from build123d import *

# Parameters (mm, degrees)
SKETCH1_W           = 75
SKETCH1_H           = 148
BOSS_EXTRUDE1_DEPTH = 10
SKETCH2_W           = 55
SKETCH2_H           = 8
BOSS_EXTRUDE2_DEPTH = 42
SKETCH3_W           = 26.5
SKETCH3_H           = 24
CUT_EXTRUDE1_DEPTH  = 8
SKETCH4_W           = 8
SKETCH4_H           = 30
SKETCH4_H_2         = 25
BOSS_EXTRUDE3_DEPTH = 42
SKETCH5_R           = 2.5
CUT_EXTRUDE2_DEPTH  = 8
CUT_EXTRUDE3_DEPTH  = 8
SKETCH10_R          = 2.75
CUT_EXTRUDE5_DEPTH  = 10
SKETCH11_W          = 47
SKETCH11_H          = 85
CUT_EXTRUDE6_DEPTH  = 10


with BuildPart() as part:
    # Sketch1 → Boss-Extrude1 (new body)
    with BuildSketch(Plane.XY):
        with Locations((27.5, -70)):
            Rectangle(SKETCH1_W, SKETCH1_H)
    extrude(amount=BOSS_EXTRUDE1_DEPTH)

    # Sketch2 → Boss-Extrude2 (add)
    with BuildSketch(Plane.XY.offset(10)):
        with Locations((37.5, -115)):
            Rectangle(SKETCH2_W, SKETCH2_H)
    extrude(amount=BOSS_EXTRUDE2_DEPTH)

    # Sketch3 → Cut-Extrude1 (cut)
    with BuildSketch(Plane(origin=(0, -119, 0), x_dir=(-1, 0, 0), z_dir=(0, -1, 0))):
        with Locations((-34.85, -31.15)):
            Rectangle(SKETCH3_W, SKETCH3_H)
    extrude(amount=-CUT_EXTRUDE1_DEPTH, mode=Mode.SUBTRACT)

    # Sketch4 → Boss-Extrude3 (add)
    with BuildSketch(Plane.XY.offset(10)):
        with Locations((61, -11)):
            Rectangle(SKETCH4_W, SKETCH4_H)
        with Locations((61, -131.5)):
            Rectangle(SKETCH4_W, SKETCH4_H_2)
    extrude(amount=BOSS_EXTRUDE3_DEPTH)

    # Sketch5 → Cut-Extrude2 (cut)
    with BuildSketch(Plane.ZY.offset(-57)):
        with Locations((18, -11)):
            Circle(SKETCH5_R)
        with Locations((44, -11)):
            Circle(SKETCH5_R)
        with Locations((44, -129)):
            Circle(SKETCH5_R)
        with Locations((18, -129)):
            Circle(SKETCH5_R)
    extrude(amount=-CUT_EXTRUDE2_DEPTH, mode=Mode.SUBTRACT)

    # Sketch6 → Cut-Extrude3 (cut)
    with BuildSketch(Plane(origin=(0, -119, 0), x_dir=(-1, 0, 0), z_dir=(0, -1, 0))):
        with BuildLine():
            Line((-19.4, -45.1), (-17.4, -45.1))
            ThreePointArc((-17.4, -45.1), (-15.85, -46.65), (-17.4, -48.2))
            Line((-17.4, -48.2), (-19.4, -48.2))
            ThreePointArc((-19.4, -48.2), (-20.95, -46.65), (-19.4, -45.1))
        make_face()
        with BuildLine():
            Line((-19.4, -14.1), (-17.4, -14.1))
            ThreePointArc((-17.4, -14.1), (-15.85, -15.65), (-17.4, -17.2))
            Line((-17.4, -17.2), (-19.4, -17.2))
            ThreePointArc((-19.4, -17.2), (-20.95, -15.65), (-19.4, -14.1))
        make_face()
        with BuildLine():
            Line((-50.4, -45.1), (-48.4, -45.1))
            ThreePointArc((-48.4, -45.1), (-46.85, -46.65), (-48.4, -48.2))
            Line((-48.4, -48.2), (-50.4, -48.2))
            ThreePointArc((-50.4, -48.2), (-51.95, -46.65), (-50.4, -45.1))
        make_face()
        with BuildLine():
            Line((-50.4, -14.1), (-48.4, -14.1))
            ThreePointArc((-48.4, -14.1), (-46.85, -15.65), (-48.4, -17.2))
            Line((-48.4, -17.2), (-50.4, -17.2))
            ThreePointArc((-50.4, -17.2), (-51.95, -15.65), (-50.4, -14.1))
        make_face()
    extrude(amount=-CUT_EXTRUDE3_DEPTH, mode=Mode.SUBTRACT)

    # Sketch10 → Cut-Extrude5 (cut)
    with BuildSketch(Plane(origin=(0, 0, 0), x_dir=(-1, 0, 0), z_dir=(0, 0, -1))):
        with Locations((-1, -102.8)):
            Circle(SKETCH10_R)
        with Locations((-1, -134.8)):
            Circle(SKETCH10_R)
        with Locations((-1, -37.7)):
            Circle(SKETCH10_R)
        with Locations((-1, -5.7)):
            Circle(SKETCH10_R)
    extrude(amount=-CUT_EXTRUDE5_DEPTH, mode=Mode.SUBTRACT)

    # Sketch11 → Cut-Extrude6 (cut)
    with BuildSketch(Plane(origin=(0, 0, 0), x_dir=(-1, 0, 0), z_dir=(0, 0, -1))):
        with Locations((-41.5, -67.5)):
            Rectangle(SKETCH11_W, SKETCH11_H)
    extrude(amount=-CUT_EXTRUDE6_DEPTH, mode=Mode.SUBTRACT)


solid = part.part
Verification items for the finished model (mm, model axes). A direction names the side the tool comes from. Coordinates: 2 decimals unless noted, no trailing zeros. Order: outer loops, then holes, each group sorted by start corner. A loop starts at its lowest first (then second) coordinate and runs counter-clockwise, first axis right, second up.
Item 1: Material ranges on L1, parallel to Y at x = 62.25, z = 44; L2, parallel to Z at x = 61, y = -129; L3, parallel to Z at x = 37, y = -124, recorded low to high.
Filled in:
L1: y = -144 to -131.5, -126.5 to -111, -26 to -13.5, -8.5 to 4
L2: z = 0 to 15.5, 20.5 to 41.5, 46.5 to 52
L3: z = 0 to 10
Item 2: Release check for a two-part mould opening along Y. For faces 1 (the face through (38, 4, 9)), 2 (the face through (20.95, -115.06, 46.68)), 3 (the face through (60.94, -11.96, 46.31)) record: +Y half, -Y half, draft (parallel to the pull), parting line (faces both ways), or undercut.
Filled in:
face 1: +Y half
face 2: draft
face 3: undercut
Item 3: Section check C-C, the plane z = 26.5. Enter the section's corners in (x, y), then the cut area to 3 significant figures.
Filled in:
outline: (10, -119) - (21.6, -119) - (21.6, -111) - (10, -111) - close; (48.1, -119) - (57, -119) - (57, -144) - (65, -144) - (65, -111) - (48.1, -111) - close; (57, -26) - (65, -26) - (65, 4) - (57, 4) - close
area: 668 mm2
Item 4: Depth check by flat-ended pin: pin 1 (2 mm diameter, centred on x = 49.5, y = -113, fed in from -Z); pin 2 (12.5 mm diameter, centred on y = -132, z = 25.5, fed in from -X); pin 3 (4 mm diameter, centred on x = 18, y = -33, fed in from +Z); pin 4 (6.5 mm diameter, centred on y = -116.5, z = 38.5, fed in from -X). Enter the tip coordinate at first touch or a pass-through.
Filled in:
pin 1: stops at z = 0
pin 2: stops at x = 57
pin 3: stops at z = 10
pin 4: stops at x = 10
Item 5: Section check A-A, the plane x = 59.5. Enter the section's corners in (y, z), then the cut area to 3 significant figures.
Filled in:
outline: (-144, 0) - (-110, 0) - (-110, 10) - (-111, 10) - (-111, 52) - (-144, 52) - close; (-26, 10) - (-25, 10) - (-25, 0) - (4, 0) - (4, 52) - (-26, 52) - close; hole circle Ø5 at (-129, 18); hole circle Ø5 at (-129, 44); hole circle Ø5 at (-11, 18); hole circle Ø5 at (-11, 44)
area: 3,200 mm2
Item 6: Section check D-D, the plane x = 1. Enter the section's corners in (y, z).
Filled in:
outline: (-144, 0) - (-137.55, 0) - (-137.55, 10) - (-144, 10) - close; (-132.05, 0) - (-105.55, 0) - (-105.55, 10) - (-132.05, 10) - close; (-100.05, 0) - (-40.45, 0) - (-40.45, 10) - (-100.05, 10) - close; (-34.95, 0) - (-8.45, 0) - (-8.45, 10) - (-34.95, 10) - close; (-2.95, 0) - (4, 0) - (4, 10) - (-2.95, 10) - close
Item 7: Section check B-B, the plane y = -102.8. Enter the section's corners in (x, z).
Filled in:
outline: (-10, 0) - (-1.75, 0) - (-1.75, 10) - (-10, 10) - close; (3.75, 0) - (18, 0) - (18, 10) - (3.75, 10) - close
Item 8: Access from +Z, -Z, +X, -X, +Y, -Y to the whole of each face (thin tool, end or side, straight path). Record for faces 4 (the face through (61, -26, 31)), 5 (the face through (57, -11, 31)), 6 (the face through (51.95, -115.06, 15.68)).
Filled in:
face 4: +Z, -Z, +X, -X
face 5: +Z, -X, +Y
face 6: +Y, -Y
